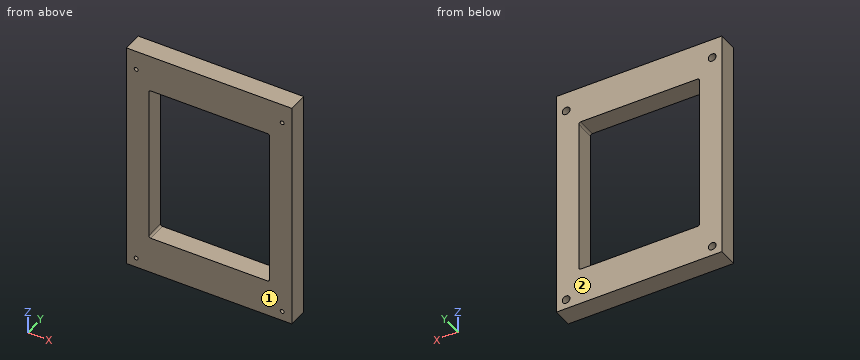
from build123d import *

# Parameters (mm, degrees)
SKETCH1_W           = 85
SKETCH1_H           = 120
BOSS_EXTRUDE1_DEPTH = 10
SKETCH2_W           = 62
SKETCH2_H           = 82
CUT_EXTRUDE1_DEPTH  = 10
FILLET1_R           = 1
SKETCH3_R           = 2
CUT_EXTRUDE2_DEPTH  = 5
SKETCH4_R           = 1
CUT_EXTRUDE3_DEPTH  = 5


with BuildPart() as part:
    # Sketch1 → Boss-Extrude1 (new body)
    with BuildSketch(Plane(origin=(0, 0, 0), x_dir=(1, 0, 0), z_dir=(0, 1, 0))):
        Rectangle(SKETCH1_W, SKETCH1_H)
    extrude(amount=BOSS_EXTRUDE1_DEPTH)

    # Sketch2 → Cut-Extrude1 (cut)
    with BuildSketch(Plane(origin=(0, 10, 0), x_dir=(1, 0, 0), z_dir=(0, 1, 0))):
        Rectangle(SKETCH2_W, SKETCH2_H)
    extrude(amount=-CUT_EXTRUDE1_DEPTH, mode=Mode.SUBTRACT)

    # Fillet1
    fillet1_edges = [part.edges().sort_by_distance(p)[0] for p in [
        (31, 5, -41),
        (31, 5, 41),
        (-31, 5, 41),
        (-31, 5, -41),
    ]]
    fillet(fillet1_edges, radius=FILLET1_R)

    # Sketch3 → Cut-Extrude2 (cut)
    with BuildSketch(Plane(origin=(0, 10, 0), x_dir=(1, 0, 0), z_dir=(0, 1, 0))):
        with Locations((-37.5, -50)):
            Circle(SKETCH3_R)
        with Locations((-37.5, 55)):
            Circle(SKETCH3_R)
        with Locations((37.5, 55)):
            Circle(SKETCH3_R)
        with Locations((37.5, -50)):
            Circle(SKETCH3_R)
    extrude(amount=-CUT_EXTRUDE2_DEPTH, mode=Mode.SUBTRACT)

    # Sketch4 → Cut-Extrude3 (cut)
    with BuildSketch(Plane(origin=(0, 5, 0), x_dir=(1, 0, 0), z_dir=(0, 1, 0))):
        with Locations((-37.5, -50)):
            Circle(SKETCH4_R)
        with Locations((37.5, -50)):
            Circle(SKETCH4_R)
        with Locations((37.5, 55)):
            Circle(SKETCH4_R)
        with Locations((-37.5, 55)):
            Circle(SKETCH4_R)
    extrude(amount=-CUT_EXTRUDE3_DEPTH, mode=Mode.SUBTRACT)


solid = part.part
Read the model definition and answer for the solid it produces. Units are mm, in the model's axes. Face numbers are marked on the shaded views. Coordinates: 2 decimals unless noted, no trailing zeros. Loops run counter-clockwise (first coordinate to the right, second up) from the corner with the lowest first, then second, coordinate; pieces in that order, holes last. Notation, with made-up numbers: (-36.5, -13.5) - (-3.5, -13.5) arc R29 cw to (-3.5, 15.5) - close; hole circle Ø4 at (-31, -26.75). An arc over 180 degrees is marked (long way). Answer in a Markdown table with one row per item.
Q1. Given P1, Ø3.5, axis at x = 37.5, z = -55, coming from the +Y side, flat-ended and moving along its own axis, determine where the tip first touches the part or whether it passes through.
Here are the results:
| item | result |
|---|---|
| P1 | stops at y = 5 |
Q2. Find section A-A on y = 8.25. Write down the section's boundary in (x, z).
Here are the results:
| item | result |
|---|---|
| outline | (-42.5, -60) - (42.5, -60) - (42.5, 60) - (-42.5, 60) - close; hole circle Ø4 at (-37.5, -55); hole circle Ø4 at (-37.5, 50); hole (-31, -40) arc R1 ccw to (-30, -41) - (30, -41) arc R1 ccw to (31, -40) - (31, 40) arc R1 ccw to (30, 41) - (-30, 41) arc R1 ccw to (-31, 40) - close; hole circle Ø4 at (37.5, -55); hole circle Ø4 at (37.5, 50) |
Q3. Find section C-C on z = -20.5. Write down the section's boundary in (x, y).
Here are the results:
| item | result |
|---|---|
| outline | (-42.5, 0) - (-31, 0) - (-31, 10) - (-42.5, 10) - close; (31, 0) - (42.5, 0) - (42.5, 10) - (31, 10) - close |
Q4. Find section B-B on x = -26. Write down the section's boundary in (y, z).
Here are the results:
| item | result |
|---|---|
| outline | (0, -60) - (10, -60) - (10, -41) - (0, -41) - close; (0, 41) - (10, 41) - (10, 60) - (0, 60) - close |
Q5. The mould has two halves that part along Y. Classify the marked faces 1 and 2: pulls with the +Y half, pulls with the -Y half, needs draft (parallel to the pull), parting line crosses it, or undercut.
Here are the results:
| item | result |
|---|---|
| face 1 | pulls with the -Y half |
| face 2 | pulls with the +Y half |
Q6. Straight lines are drawn through the part: line 1 along Z through (x, y) = (-37.5, 3.8); line 2 along X through (y, z) = (8.55, 50); line 3 along Z through (x, y) = (-24, 3). For each, find the intervals that lie inside material, in ascending order. Write a range as [from, to].
Here are the results:
| item | result |
|---|---|
| line 1 | z = [-60, -56], [-54, 49], [51, 60] |
| line 2 | x = [-42.5, -39.5], [-35.5, 35.5], [39.5, 42.5] |
| line 3 | z = [-60, -41], [41, 60] |
